Can you work these out from the model? Positions are in its coordinate system, mm. A direction names the side the tool comes from. Coordinates: 2 decimals unless noted, no trailing zeros. Loops run counter-clockwise (first coordinate to the right, second up) from the corner with the lowest first, then second, coordinate; pieces in that order, holes last.
```python
from build123d import *

# Parameters (mm, degrees)
F0_R     = 1.1684
F1_DEPTH = 1.1811
F3_DEPTH = 4.953
F5_DEPTH = 3.5814
F7_DEPTH = 4.4069


with BuildPart() as f1:
    # F0 (on Top) → F1 (new body, symmetric)
    with BuildSketch(Plane.XY):
        with BuildLine():
            Line((17.2847, 3.9116), (-17.2847, 3.9116))
            ThreePointArc((-17.2847, 3.9116), (-18.398252, 3.450352), (-18.8595, 2.3368))
            Line((-18.8595, 2.3368), (-18.8595, -2.3368))
            ThreePointArc((-18.8595, -2.3368), (-18.398252, -3.450352), (-17.2847, -3.9116))
            Line((-17.2847, -3.9116), (17.2847, -3.9116))
            ThreePointArc((17.2847, -3.9116), (18.398252, -3.450352), (18.8595, -2.3368))
            Line((18.8595, -2.3368), (18.8595, 2.3368))
            ThreePointArc((18.8595, 2.3368), (18.398252, 3.450352), (17.2847, 3.9116))
        make_face()
        with Locations((-16.0655, 0)):
            Circle(F0_R, mode=Mode.SUBTRACT)
        with Locations((16.0655, 0)):
            Circle(F0_R, mode=Mode.SUBTRACT)
    extrude(amount=F1_DEPTH, both=True)

    # F2 (on face) → F3 (join)
    with BuildSketch(Plane.XY.offset(1.1811)):
        with BuildLine():
            Line((-11.74102, -2.3368), (11.742478, -2.3368))
            ThreePointArc((11.742478, -2.3368), (13.099371, -1.561271), (13.119829, 0.001478))
            Line((13.119829, 0.001478), (12.275062, 1.525478))
            ThreePointArc((12.275062, 1.525478), (11.696982, 2.118894), (10.897711, 2.3368))
            Line((10.897711, 2.3368), (-10.896253, 2.3368))
            ThreePointArc((-10.896253, 2.3368), (-11.695525, 2.118894), (-12.273604, 1.525478))
            Line((-12.273604, 1.525478), (-13.118371, 0.001478))
            ThreePointArc((-13.118371, 0.001478), (-13.097914, -1.561271), (-11.74102, -2.3368))
        make_face()
    extrude(amount=F3_DEPTH)

    # F4 (on face) → F5 (join)
    with BuildSketch(Plane(origin=(0, 0, -1.1811), x_dir=(1, 0, 0), z_dir=(0, 0, -1))):
        with BuildLine():
            Line((12.3952, 3.175), (-12.3952, 3.175))
            ThreePointArc((-12.3952, 3.175), (-13.508752, 2.713752), (-13.97, 1.6002))
            Line((-13.97, 1.6002), (-13.97, -1.6002))
            ThreePointArc((-13.97, -1.6002), (-13.508752, -2.713752), (-12.3952, -3.175))
            Line((-12.3952, -3.175), (12.3952, -3.175))
            ThreePointArc((12.3952, -3.175), (13.508752, -2.713752), (13.97, -1.6002))
            Line((13.97, -1.6002), (13.97, 1.6002))
            ThreePointArc((13.97, 1.6002), (13.508752, 2.713752), (12.3952, 3.175))
        make_face()
    extrude(amount=F5_DEPTH)

    # F6 (on face) → F7 (join)
    with BuildSketch(Plane.XY.offset(6.1341)):
        with BuildLine():
            Line((10.710689, 2.0193), (-10.709231, 2.0193))
            ThreePointArc((-10.709231, 2.0193), (-11.508503, 1.801394), (-12.086582, 1.207978))
            Line((-12.086582, 1.207978), (-12.830227, -0.133592))
            ThreePointArc((-12.830227, -0.133592), (-12.813729, -1.393874), (-11.71946, -2.0193))
            Line((-11.71946, -2.0193), (11.720917, -2.0193))
            ThreePointArc((11.720917, -2.0193), (12.815186, -1.393874), (12.831684, -0.133592))
            Line((12.831684, -0.133592), (12.08804, 1.207978))
            ThreePointArc((12.08804, 1.207978), (11.50996, 1.801394), (10.710689, 2.0193))
        make_face()
    extrude(amount=F7_DEPTH)


solid = f1.part
```
Item 1: I'm going to push flat-ended pins straight in: P1, Ø2, axis at x = 12.5, z = 3.5, coming from the -Y side; P2, Ø3.5, axis at x = -16.07, y = 0, coming from the -Z side; P3, Ø1.5, axis at x = -3, z = 2.5, coming from the +Y side; P4, Ø1.9, axis at x = 16.07, y = 0, coming from the -Z side. Where does each tip first touch, or does it pass through?
Results are:
P1: stops at y = -2.34
P2: stops at z = -1.18
P3: stops at y = 2.34
P4: passes through
Item 2: I need wall thicknesses on line 1 along Y through (x, z) = (0, -2.25) (3 decimals); line 2 along Y through (x, z) = (2.5, 1.5); line 3 along Z through (x, y) = (-1, 3.75). Which ranges of each line are inside material? Lowest first, please.
Results are:
line 1: y = -3.175 to 3.175
line 2: y = -2.34 to 2.34
line 3: z = -1.18 to 1.18
Item 3: We'd pull the mould along Y, two halves only. Please class faces 6 (the face through (-17.233, 0.051, -0.017)), 7 (the face through (-13.496, -2.726, -2.947)), 8 (the face through (-13.52, 2.7, -2.95)), 9 (the face through (13.09, -1.58, 3.62)): +Y half, -Y half, draft (parallel to the pull), parting line (faces both ways), or undercut.
Results are:
face 6: undercut
face 7: -Y half
face 8: +Y half
face 9: parting line
Item 4: Suppose I cut it at D-D, the plane y = 2.75. Please give me the cut outline in (x, z), plus the area to 3 significant figures.
Results are:
outline: (-18.8, -1.18) - (-13.47, -1.18) - (-13.47, -4.76) - (13.47, -4.76) - (13.47, -1.18) - (18.8, -1.18) - (18.8, 1.18) - (-18.8, 1.18) - close
area: 185 mm2
Item 5: Suppose I cut it at B-B, the plane z = 8. Please give me the cut outline in (x, y).
Results are:
outline: (-12.83, -0.13) arc R1.27 ccw to (-11.72, -2.02) - (11.72, -2.02) arc R1.27 ccw to (12.83, -0.13) - (12.09, 1.21) arc R1.57 ccw to (10.71, 2.02) - (-10.71, 2.02) arc R1.57 ccw to (-12.09, 1.21) - close
Item 6: Suppose I cut it at C-C, the plane x = 16. Please give me the cut outline in (y, z), plus the area to 3 significant figures.
Results are:
outline: (-3.91, -1.18) - (-1.17, -1.18) - (-1.17, 1.18) - (-3.91, 1.18) - close; (1.17, -1.18) - (3.91, -1.18) - (3.91, 1.18) - (1.17, 1.18) - close
area: 13.0 mm2
Item 7: On a 3-axis mill with a long thin cutter (end or side, diameter ignored), from which of +Z, -Z, +X, -X, +Y, -Y can I reach the whole of each face in a straight line? I mean faces 1 (the face through (-13.11, -1.54, 3.62)), 2 (the face through (0, -2.337, 4)), 3 (the face through (12.465, 0.528, 8.307)), 4 (the face through (0, 2.019, 8)), 5 (the face through (13.97, 0, -3)). Say none if no direction works.
Results are:
face 1: +Z, -X
face 2: +Z, +X, -X, -Y
face 3: +Z, +X, +Y
face 4: +Z, +X, -X, +Y
face 5: -Z, +X, +Y, -Y
